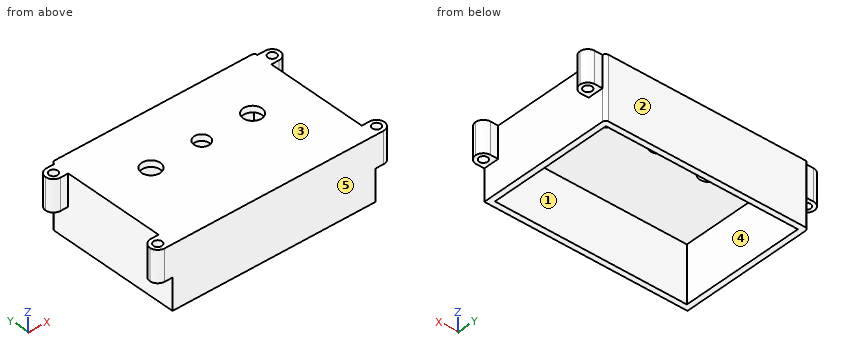
Autodesk Inventor part; units mm, degrees
ref_plane "YZ Plane" through (0, 0, 0) normal (1, 0, 0) x (0, 1, 0)
ref_plane "XZ Plane" through (0, 0, 0) normal (0, 1, 0) x (-1, 0, 0)
ref_plane "XY Plane" through (0, 0, 0) normal (0, 0, 1) x (1, 0, 0)
sketch "Sketch1" plane through (0, 0, 0) normal (0, 0, 1) x (1, 0, 0)
  line L0 (0, 0) -> (-65, 0)
  line L1 (-65, 0) -> (-65, 43.5)
  line L2 (-65, 43.5) -> (0, 43.5)
  line L3 (0, 43.5) -> (0, 0)
  dimension "d0" = 43.5
  dimension "d1" = 65
extrude "Extrusion1" add sketch "Sketch1" along normal blind 20
sketch "Sketch2" plane through (0, 0, 0) normal (0, 0, -1) x (-1, 0, 0)
  line L0 (1.8, 41.7) -> (63.2, 41.7)
  line L1 (63.2, 41.7) -> (63.2, 1.8)
  line L2 (63.2, 1.8) -> (1.8, 1.8)
  line L3 (1.8, 1.8) -> (1.8, 41.7)
  line L4 (65, 43.5) -> (65, 0)
  line L5 (0, 43.5) -> (65, 43.5)
  line L6 (0, 0) -> (0, 43.5)
  line L7 (65, 0) -> (0, 0)
  point P0 (65, 21.75)
  dimension "d4" = 1.8
  dimension "d5" = 1.8
  dimension "d6" = 1.8
  dimension "d7" = 1.8
extrude "Extrusion2" cut sketch "Sketch2" against normal blind 18 contours L0 L1 L2 L3
sketch "Sketch3" plane through (0, 0, 20) normal (0, 0, 1) x (1, 0, 0)
  circle A0 centre (-48.75, 26) radius 3
  circle A1 centre (-32.5, 26) radius 2.5
  circle A2 centre (-16.25, 26) radius 3
  line L0 (-65, 43.5) -> (-65, 0)
  line L1 (0, 43.5) -> (-65, 43.5)
  point P0 (0, 0)
  dimension "d10" = 16.25
  dimension "d11" = 16.25
  dimension "d12" = 16.25
  dimension "d13" = 6
  dimension "d14" = 17.5
  dimension "d15" = 5
extrude "Extrusion3" cut sketch "Sketch3" against normal up to surface (2 mm away)
fillet "Fillet1" radius 1 2 edges at (-65, 43.5, 10) (0, 43.5, 10)
sketch "Sketch4" plane through (0, 0, 20) normal (0, 0, 1) x (1, 0, 0)
  line L0 (0, 0) -> (0, 42.5)
  line L1 (0, 42.5) -> (5, 42.5)
  line L2 (5, 42.5) -> (5, 37.5)
  line L3 (5, 37.5) -> (0, 37.5)
  line L4 (0, 37.5) -> (0, 42.5)
  line L5 (-65, 42.5) -> (-65, 0)
  line L6 (-65, 42.5) -> (-70, 42.5)
  line L7 (-70, 42.5) -> (-70, 37.5)
  line L8 (-70, 37.5) -> (-65, 37.5)
  line L9 (-65, 37.5) -> (-65, 42.5)
  circle A0 centre (-67.5, 40) radius 1.35
  circle A1 centre (2.5, 40) radius 1.35
  line L10 (0, 0) -> (5, 0)
  line L11 (5, 0) -> (5, 5)
  line L12 (5, 5) -> (0, 5)
  line L13 (0, 5) -> (0, 0)
  line L14 (-65, 0) -> (0, 0)
  line L15 (-65, 0) -> (-70, 0)
  line L16 (-70, 0) -> (-70, 5)
  line L17 (-70, 5) -> (-65, 5)
  line L18 (-65, 5) -> (-65, 0)
  circle A2 centre (-67.5, 2.5) radius 1.35
  circle A3 centre (2.5, 2.5) radius 1.35
  dimension "d19" = 5
  dimension "d20" = 5
  dimension "d21" = 5
  dimension "d22" = 5
  dimension "d23" = 2.7
  dimension "d24" = 2.7
  dimension "d25" = 5
  dimension "d26" = 5
  dimension "d27" = 5
  dimension "d28" = 5
  dimension "d29" = 2.5
  dimension "d30" = 2.5
  dimension "d31" = 2.5
  dimension "d32" = 2.5
  dimension "d33" = 2.5
  dimension "d34" = 2.5
  dimension "d35" = 2.7
  dimension "d36" = 2.7
  dimension "d37" = 2.5
  dimension "d38" = 2.5
extrude "Extrusion4" add sketch "Sketch4" against normal blind 10
full round fillet "Full Round Fillet1" first side at (3.3333, 5, 16.6667) centre faces at (5, 1.6667, 16.6667) second side at (-43.3333, 0, 16.6667)
full round fillet "Full Round Fillet2" first side at (-44.1666, 0, 16.6667) centre faces at (-70, 3.3333, 16.6667) second side at (-66.6667, 5, 16.6667)
full round fillet "Full Round Fillet3" first side at (-66.6667, 42.5, 16.6667) centre faces at (-70, 40.8333, 16.6667) second side at (-68.3333, 37.5, 16.6667)
full round fillet "Full Round Fillet4" first side at (1.6667, 37.5, 16.6667) centre faces at (5, 39.1667, 16.6667) second side at (3.3333, 42.5, 16.6667)
properties part number "BUTTON COVER"
The model under review builds one solid part; all positions refer to its coordinate system, in mm. Face numbers are marked on the shaded views. A direction names the side the tool comes from. Give positions to 0.01 mm unless a question says otherwise; leave off trailing zeros. Write each loop counter-clockwise with the first axis right and the second up, starting at its lowest first coordinate (ties: lowest second). Pieces come first, ordered by that corner, then holes.
1. For P1, Ø2, axis at x = -66.5, z = 16.5, coming from the +Y side; P2, Ø1.5, axis at x = -68, y = 1.5, coming from the -Z side; P3, Ø1.5, axis at y = 33.5, z = 7.5, coming from the -X side, all flat-tipped, find the tip position at first contact; note any pin that passes through.
2. Draft analysis for pull direction Y (two halves, no side actions). For the marked faces 3, 4 and 5, state which applies: +Y half, -Y half, draft (parallel to the pull), parting line (faces both ways), or undercut.
3. Add section C-C, the plane y = 26. Write out the cut boundary in (x, z), plus the area to 3 significant figures.
4. Add section B-B, the plane z = 18.75. Count the separate pieces of the cut face and the enclosed holes in it, plus the area to 3 significant figures.
5. Add section A-A, the plane x = -16.25. Write out the cut boundary in (y, z).
6. Add section D-D, the plane z = 6.5. Write out the cut boundary in (x, y), plus the area to 3 significant figures.
7. Tool access review of the marked faces 1 and 2: name each direction out of +Z, -Z, +X, -X, +Y, -Y from which nothing blocks a thin tool from reaching the whole face with its end or side.
8. Wall thickness on L1, parallel to Y at x = -67.5, z = 18; L2, parallel to X at y = 22, z = 12; L3, parallel to Y at x = -16.25, z = 18.7: over which ranges is each line inside the solid? List them lowest first.
Worked answers:
1. P1: stops at y = 42.5
1. P2: stops at z = 10
1. P3: stops at x = -65
2. face 3: draft
2. face 4: undercut
2. face 5: -Y half
3. outline: (-65, 0) - (-63.2, 0) - (-63.2, 18) - (-51.75, 18) - (-51.75, 20) - (-65, 20) - close; (-45.75, 18) - (-35, 18) - (-35, 20) - (-45.75, 20) - close; (-30, 18) - (-19.25, 18) - (-19.25, 20) - (-30, 20) - close; (-13.25, 18) - (-1.8, 18) - (-1.8, 0) - (0, 0) - (0, 20) - (-13.25, 20) - close
3. area: 161 mm2
4. separate pieces: 1
4. enclosed holes: 7
4. area: 2,820 mm2
5. outline: (0, 0) - (1.8, 0) - (1.8, 18) - (23, 18) - (23, 20) - (0, 20) - close; (29, 18) - (41.7, 18) - (41.7, 0) - (43.5, 0) - (43.5, 20) - (29, 20) - close
6. outline: (-65, 0) - (0, 0) - (0, 42.5) arc R1 ccw to (-1, 43.5) - (-64, 43.5) arc R1 ccw to (-65, 42.5) - close; hole (-63.2, 1.8) - (-1.8, 1.8) - (-1.8, 41.7) - (-63.2, 41.7) - close
6. area: 377 mm2
7. face 1: -Z
7. face 2: +Z, -Z, +X, -X, +Y
8. L1: y = 0 to 1.15, 3.85 to 5, 37.5 to 38.65, 41.35 to 42.5
8. L2: x = -65 to -63.2, -1.8 to 0
8. L3: y = 0 to 23, 29 to 43.5
